```python
from build123d import *

# Parameters (mm, degrees)
F0_W     = 203.2
F0_H     = 76.2
F0_R     = 1.99898
F0_R_2   = 19.05
F1_DEPTH = 12.7
F2_R     = 3.175
F3_DEPTH = 12.701


with BuildPart() as f1:
    # F0 (on Top) → F1 (new body)
    with BuildSketch(Plane.XY):
        Rectangle(F0_W, F0_H)
        with Locations((-23.749, -23.9014)):
            Circle(F0_R, mode=Mode.SUBTRACT)
        with Locations((0, -0.3302)):
            Circle(F0_R_2, mode=Mode.SUBTRACT)
        with Locations((23.3934, -23.9014)):
            Circle(F0_R, mode=Mode.SUBTRACT)
        with Locations((-23.749, 23.241)):
            Circle(F0_R, mode=Mode.SUBTRACT)
        with Locations((23.3934, 23.241)):
            Circle(F0_R, mode=Mode.SUBTRACT)
    extrude(amount=F1_DEPTH)

    # F2 (on face) → F3 (cut, through all)
    with BuildSketch(Plane.XY.offset(12.7)):
        with Locations((-88.9, -31.75)):
            Circle(F2_R)
        with Locations((-50.8, -31.75)):
            Circle(F2_R)
        with Locations((-12.7, -31.75)):
            Circle(F2_R)
        with Locations((12.7, -31.75)):
            Circle(F2_R)
        with Locations((50.8, -31.75)):
            Circle(F2_R)
        with Locations((88.9, -31.75)):
            Circle(F2_R)
    extrude(amount=-F3_DEPTH, mode=Mode.SUBTRACT)


solid = f1.part
```
The listing builds one solid part. Answer for the finished solid, in the listing's coordinates (mm). Round coordinates to 2 decimals unless told otherwise and drop trailing zeros. Order: outer loops, then holes, each group sorted by start corner. A loop starts at its lowest first (then second) coordinate and runs counter-clockwise, first axis right, second up. Notation, with made-up numbers: (22.25, -15.5) - (27.25, -15.5) arc R19 cw to (27.25, 1.5) - close; hole circle Ø2 at (23.5, -29.5). An arc over 180 degrees is marked (long way). Put each result on its own line as item: value. Start each with the question number.
(1) Find section C-C (z = 10). State how many separate pieces and enclosed holes the cut face has, plus the area to 3 significant figures.
(2) Determine the mould class of faces 1 (the cylindrical face through (18.17, 5.39, 6.26)), 2 (the flat face through (-1, -38.1, 6)), 3 (the flat face through (-24, 1, 0)) for opening direction Y: released by +Y, released by -Y, zero draft, split by the parting line, or undercut.
(3) Find section B-B (y = 16). Give the vertices of the cut face in (x, z), plus the area to 3 significant figures.
(4) Straight lines are drawn through the part: probe 1 along Y at (x, z) = (23.5, 8); probe 2 along X at (y, z) = (24, 8.25); probe 3 along Y at (x, z) = (88.9, 9.5) (3 decimals). For each, find the intervals that lie inside material, in ascending order. Write a range as from..to.
(5) Find section A-A (x = 0). Give the vertices of the cut face in (y, z), plus the area to 3 significant figures.
Reply:
1. separate pieces: 1
1. enclosed holes: 11
1. area: 14,100 mm^2
2. face 1: undercut
2. face 2: released by -Y
2. face 3: zero draft
3. outline: (-101.6, 0) - (-9.81, 0) - (-9.81, 12.7) - (-101.6, 12.7) - close; (9.81, 0) - (101.6, 0) - (101.6, 12.7) - (9.81, 12.7) - close
3. area: 2,330 mm^2
4. probe 1: -38.1..-25.9, -21.91..21.24, 25.24..38.1
4. probe 2: -101.6..-25.6, -21.9..21.54, 25.24..101.6
4. probe 3: -38.1..-34.925, -28.575..38.1
5. outline: (-38.1, 0) - (-19.38, 0) - (-19.38, 12.7) - (-38.1, 12.7) - close; (18.72, 0) - (38.1, 0) - (38.1, 12.7) - (18.72, 12.7) - close
5. area: 484 mm^2
